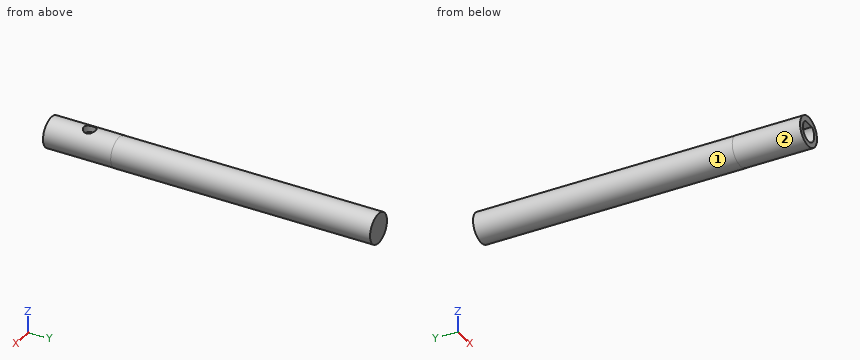
from build123d import *

# Parameters (mm, degrees)
SKETCH1_R               = 3.75
BOSS_EXTRUDE1_DEPTH     = 17
SKETCH2_R               = 3.75
SKETCH2_R_2             = 0.058819456
BOSS_EXTRUDE2_DEPTH     = 65
CUT_EXTRUDE1_REACH      = 84.174
CUT_EXTRUDE1_END_RADIUS = 3.75
SKETCH3_R               = 1.5


with BuildPart() as part:
    # Sketch1 → Boss-Extrude1 (new body)
    with BuildSketch(Plane(origin=(0, 0, 0), x_dir=(1, 0, 0), z_dir=(0, 1, 0))):
        with Locations(Location((0, 0, 0), (0, 0, 270))):
            Circle(SKETCH1_R)
        with BuildLine():
            Line((1.5, -2), (-1.5, -2))
            ThreePointArc((-1.5, -2), (0, 2.5), (1.5, -2))
        make_face(mode=Mode.SUBTRACT)
    extrude(amount=BOSS_EXTRUDE1_DEPTH)

    # Sketch2 → Boss-Extrude2 (add)
    with BuildSketch(Plane(origin=(0, 17, 0), x_dir=(1, 0, 0), z_dir=(0, 1, 0))):
        with Locations(Location((0.058819456, 0, 0), (0, 0, 90.449352147))):
            Circle(SKETCH2_R)
        with Locations(Location((0.058819456, 0, 0), (0, 0, 270))):
            Circle(SKETCH2_R_2, mode=Mode.SUBTRACT)
    extrude(amount=BOSS_EXTRUDE2_DEPTH)

    # Cut-Extrude1: up to this cylinder (the profile starts inside it)
    cut_extrude1_end = Plane(origin=(0, 9.674653, 0), z_dir=(0, -1, 0)) * Cylinder(CUT_EXTRUDE1_END_RADIUS, 176.848, mode=Mode.PRIVATE)
    # Sketch3 → Cut-Extrude1 (cut, up to the surface)
    with BuildSketch(Plane.XY, mode=Mode.PRIVATE) as cut_extrude1_sk1:
        with Locations(Location((0.177976735, 9.674652852, 0), (0, 0, 180))):
            Circle(SKETCH3_R)
    cut_extrude1_tool1 = extrude(cut_extrude1_sk1.sketch, amount=CUT_EXTRUDE1_REACH, mode=Mode.PRIVATE) & cut_extrude1_end
    add(cut_extrude1_tool1.solids().sort_by_distance((0.177977, 9.674653, 0))[0], mode=Mode.SUBTRACT)


solid = part.part
Input: part model. Units: mm. Frame: model coordinates. Face numbers are marked on the shaded views. A direction names the side the tool comes from. Round coordinates to 2 decimals unless told otherwise and drop trailing zeros. Order: outer loops, then holes, each group sorted by start corner. A loop starts at its lowest first (then second) coordinate and runs counter-clockwise, first axis right, second up.
1. Set-up query: the marked faces 1 and 2. Return all of +Z, -Z, +X, -X, +Y, -Y with unobstructed straight access to the full face (end or side cutting, diameter ignored); none if empty.
The answers:
face 1: +Y
face 2: -Y
2. Cut plane A-A, the plane y = 40. Output: boundary loops of the cut face in (x, z).
The answers:
outline: circle Ø7.5 at (0.06, 0); hole circle Ø0.12 at (0.06, 0)
3. Pin query (flat end, axial travel): P1, Ø2, axis at x = 0, z = -1, coming from the -Y side; P2, Ø3, axis at y = 59.5, z = 2.5, coming from the +X side; P3, Ø1, axis at x = -3, y = 24, coming from the +Z side. Return the tip coordinate at first contact, or that it passes through.
The answers:
P1: stops at y = 17
P2: stops at x = 3.67
P3: stops at z = 2.74
4. Material intervals for line 1 (X direction, y = 7.5, z = 0); line 2 (Z direction, x = 0, y = 11.5); line 3 (Y direction, x = 0.25, z = 3.25), sorted ascending.
The answers:
line 1: x = -3.75 to -2.5, 2.5 to 3.75
line 2: z = -3.75 to -2.5, 2 to 3.75
line 3: y = 0 to 8.18, 11.17 to 82
